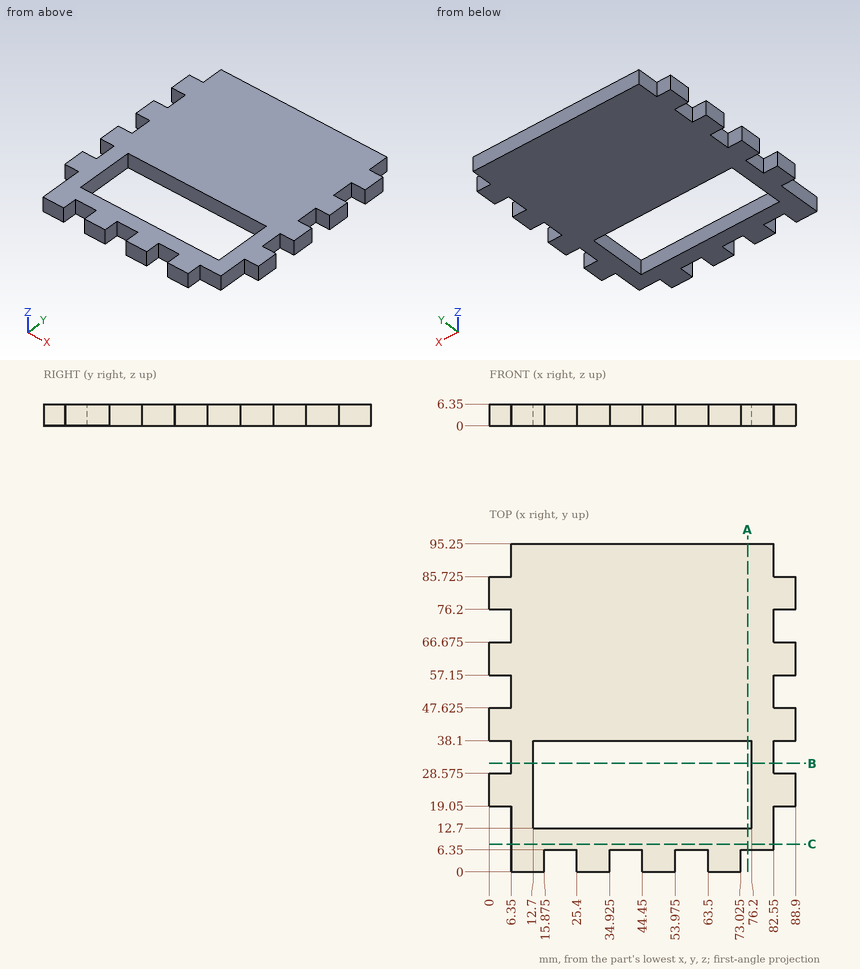
The figure shows three views and two pictorial views of one solid part (mm, origin at its lowest corner). Answer the questions. Coordinates: 2 decimals unless noted, no trailing zeros. Loops run counter-clockwise (first coordinate to the right, second up) from the corner with the lowest first, then second, coordinate; pieces in that order, holes last.
(1) The part is cut by section A-A (x = 75). Determine the outline of the cut face in (y, z).
Solution:
outline: (6.35, 0) - (12.7, 0) - (12.7, 6.35) - (6.35, 6.35) - close; (38.1, 0) - (95.25, 0) - (95.25, 6.35) - (38.1, 6.35) - close
(2) Flat-ended cylindrical pins translate along their axes: pin 1 Ø1.9 at (y, z) = (30, 4.5) entering from +X; pin 2 Ø3 at (x, z) = (58, 4) entering from -Y; pin 3 Ø3 at (x, z) = (85, 3) entering from +Y (3 decimals). Find the tip coordinate at first contact, or state that the pin passes through.
Solution:
pin 1: stops at x = 82.55
pin 2: stops at y = 6.35
pin 3: stops at y = 85.725
(3) The part is cut by section B-B (y = 31.5). Determine the outline of the cut face in (x, z), and give its area (3 significant figures).
Solution:
outline: (6.35, 0) - (12.7, 0) - (12.7, 6.35) - (6.35, 6.35) - close; (76.2, 0) - (82.55, 0) - (82.55, 6.35) - (76.2, 6.35) - close
area: 80.6 mm2
(4) The part is cut by section C-C (y = 8). Determine the outline of the cut face in (x, z).
Solution:
outline: (6.35, 0) - (82.55, 0) - (82.55, 6.35) - (6.35, 6.35) - close
(5) Consider line 1 along Y through (x, z) = (59.5, 1.25); line 2 along Y through (x, z) = (31, 3.5); line 3 along X through (y, z) = (14, 5). Determine where each line is inside the solid, lowest interval first.
Solution:
line 1: y = 6.35 to 12.7, 38.1 to 95.25
line 2: y = 0 to 12.7, 38.1 to 95.25
line 3: x = 6.35 to 12.7, 76.2 to 82.55
